from build123d import *

# Parameters (mm, degrees)
PAD005_DEPTH                  = 17
PAD006_DEPTH                  = 4.5
SKETCH015_R                   = 2.75
POCKET005_DEPTH               = 93.84909
SKETCH016_R                   = 5
POCKET006_DEPTH               = 16.5
PAD005_MIRRORED002_2_DEPTH    = 17
PAD006_MIRRORED002_2_DEPTH    = 4.5
SKETCH015_MIRRORED002_2_R     = 2.75
POCKET005_MIRRORED002_2_DEPTH = 93.84909
SKETCH016_MIRRORED002_2_R     = 5
POCKET006_MIRRORED002_2_DEPTH = 16.5
SKETCH023_W                   = 1
SKETCH023_H                   = 10
POCKET011_DEPTH               = 0.2


with BuildPart() as part:
    # Sketch013 → Pad005 (new body)
    with BuildSketch(Plane.YZ):
        with BuildLine():
            ThreePointArc((0, -13.5), (4.330629, -12.786542), (8.203522, -10.721578))
            ThreePointArc((10.083563, -12.5), (9.900722, -10.810344), (8.203522, -10.721578))
            Line((6, -18.5), (10.083563, -12.5))
            Line((0, -18.5), (6, -18.5))
            Line((0, -13.5), (0, -18.5))
        make_face()
    pad005 = extrude(amount=PAD005_DEPTH)

    # Sketch014 → Pad006 (join)
    with BuildSketch(Plane.YZ.offset(17)):
        with BuildLine():
            ThreePointArc((0, -10.15), (8.790158, -5.075), (8.790158, 5.075))
            ThreePointArc((12.773875, 11.975), (8.790158, 9.675), (8.790158, 5.075))
            ThreePointArc((12.773875, 9.125), (14.198875, 10.55), (12.773875, 11.975))
            ThreePointArc((12.773875, 9.125), (11.25833, 8.25), (11.25833, 6.5))
            ThreePointArc((12.442941, -3.764734), (12.914285, 1.490384), (11.25833, 6.5))
            Line((12.442941, -3.764734), (9.8, -12.5))
            Line((9.8, -12.5), (0, -14.15))
            Line((0, -10.15), (0, -14.15))
        make_face()
    pad006 = extrude(amount=-PAD006_DEPTH)

    # Sketch015 → Pocket005 (cut, through all)
    with BuildSketch(Plane.XY):
        Circle(SKETCH015_R)
    pocket005 = extrude(amount=-POCKET005_DEPTH, mode=Mode.SUBTRACT)

    # Sketch016 → Pocket006 (cut)
    with BuildSketch(Plane.XY):
        Circle(SKETCH016_R)
    pocket006 = extrude(amount=-POCKET006_DEPTH, mode=Mode.SUBTRACT)

    # Sketch013 Mirrored002 2 → Pad005 Mirrored002 2 (add)
    with BuildSketch(Plane(origin=(0, 0, 0), x_dir=(0, -1, 0), z_dir=(-1, 0, 0))):
        with BuildLine():
            ThreePointArc((0, -13.5), (4.330629, -12.786542), (8.203522, -10.721578))
            ThreePointArc((10.083563, -12.5), (9.900722, -10.810344), (8.203522, -10.721578))
            Line((6, -18.5), (10.083563, -12.5))
            Line((0, -18.5), (6, -18.5))
            Line((0, -13.5), (0, -18.5))
        make_face()
    pad005_mirrored002_2 = extrude(amount=-PAD005_MIRRORED002_2_DEPTH)

    # Sketch014 Mirrored002 2 → Pad006 Mirrored002 2 (add)
    with BuildSketch(Plane(origin=(17, 0, 0), x_dir=(0, -1, 0), z_dir=(-1, 0, 0))):
        with BuildLine():
            ThreePointArc((0, -10.15), (8.790158, -5.075), (8.790158, 5.075))
            ThreePointArc((12.773875, 11.975), (8.790158, 9.675), (8.790158, 5.075))
            ThreePointArc((12.773875, 9.125), (14.198875, 10.55), (12.773875, 11.975))
            ThreePointArc((12.773875, 9.125), (11.25833, 8.25), (11.25833, 6.5))
            ThreePointArc((12.442941, -3.764734), (12.914285, 1.490384), (11.25833, 6.5))
            Line((12.442941, -3.764734), (9.8, -12.5))
            Line((9.8, -12.5), (0, -14.15))
            Line((0, -10.15), (0, -14.15))
        make_face()
    pad006_mirrored002_2 = extrude(amount=PAD006_MIRRORED002_2_DEPTH)

    # Sketch015 Mirrored002 2 → Pocket005 Mirrored002 2 (cut, through all)
    with BuildSketch(Plane(origin=(0, 0, 0), x_dir=(1, 0, 0), z_dir=(0, 0, -1))):
        Circle(SKETCH015_MIRRORED002_2_R)
    pocket005_mirrored002_2 = extrude(amount=POCKET005_MIRRORED002_2_DEPTH, mode=Mode.SUBTRACT)

    # Sketch016 Mirrored002 2 → Pocket006 Mirrored002 2 (cut)
    with BuildSketch(Plane(origin=(0, 0, 0), x_dir=(1, 0, 0), z_dir=(0, 0, -1))):
        Circle(SKETCH016_MIRRORED002_2_R)
    pocket006_mirrored002_2 = extrude(amount=POCKET006_MIRRORED002_2_DEPTH, mode=Mode.SUBTRACT)

    # Mirrored003: Pad005, Pad006, Pocket005, Pocket006, Pad005 Mirrored002 2, Pad006 Mirrored002 2, Pocket005 Mirrored002 2, Pocket006 Mirrored002 2 across YZ
    add(pad005.mirror(Plane.YZ))
    add(pad006.mirror(Plane.YZ))
    add(pocket005.mirror(Plane.YZ), mode=Mode.SUBTRACT)
    add(pocket006.mirror(Plane.YZ), mode=Mode.SUBTRACT)
    add(pad005_mirrored002_2.mirror(Plane.YZ))
    add(pad006_mirrored002_2.mirror(Plane.YZ))
    add(pocket005_mirrored002_2.mirror(Plane.YZ), mode=Mode.SUBTRACT)
    add(pocket006_mirrored002_2.mirror(Plane.YZ), mode=Mode.SUBTRACT)

    # Sketch023 → Pocket011 (cut)
    with BuildSketch(Plane.YZ.offset(29)):
        with Locations((0, -15)):
            Rectangle(SKETCH023_W, SKETCH023_H)
    pocket011 = extrude(amount=-POCKET011_DEPTH, mode=Mode.SUBTRACT)

    # Mirrored006: Pocket011 across YZ
    add(pocket011.mirror(Plane.YZ), mode=Mode.SUBTRACT)


solid = part.part
Build history of the part. All positions in model axes, mm. A direction names the side the tool comes from. Coordinates: 2 decimals unless noted, no trailing zeros. Order: outer loops, then holes, each group sorted by start corner. A loop starts at its lowest first (then second) coordinate and runs counter-clockwise, first axis right, second up. Notation, with made-up numbers: (71.25, -17.5) - (106.25, -17.5) arc R20 ccw to (106.25, -7.5) - close; hole circle Ø7 at (69.25, 3.5). An arc over 180 degrees is marked (long way). Write each question's results on one line, items separated by ' | '. Start each with the question number.
Item 1: Tool access for faces 4 (the face through (0.24, -9.92, -10.83)), 5 (the face through (-2.685, 0.596, -17.486)), 6 (the face through (14.782, 8.824, 9.733)), 7 (the face through (-12.5, -6.4, -8.3)): list every direction of +Z, -Z, +X, -X, +Y, -Y with a clear straight run to the whole face (end or side of a thin tool).
Item 2: Band-saw the part on A-A on x = 11. Write the cut outline in (y, z).
Item 3: Band-saw the part on D-D on z = 4.5. Write the cut outline in (x, y), and give its area (3 significant figures).
Item 4: Wall check: probe 1 along X at (y, z) = (0, -13.75); probe 2 along X at (y, z) = (9, -8); probe 3 along Z at (x, y) = (8.5, 0.5). Give the ranges that are in metal, low to high. Write a range as [from, to].
Item 5: Band-saw the part on B-B on z = -6. Write the cut outline in (x, y).
Item 6: Band-saw the part on C-C on y = 7.5. Write the cut outline in (x, z).
Item 7: Mould opens along Z. For faces 1 (the face through (0.238, -8.013, -15.542)), 2 (the face through (12.5, -6.4, -8.3)), 3 (the face through (14.782, -12.923, 1.416)) say: released by +Z, released by -Z, zero draft, split by the parting line, or undercut.
Item 8: Flat gauge pins, fed straight in: pin 1 (6 mm diameter, centred on x = -13, z = -2.5, fed in from +Y); pin 2 (3 mm diameter, centred on x = -2, y = 0.5, fed in from +Z); pin 3 (5.5 mm diameter, centred on x = -3, y = -3, fed in from +Z). Where does each tip first touch, or does it go through?
Numbers:
1) face 4: none | face 5: +Z, -Z | face 6: +X, -X | face 7: +Z
2) outline: (-10.08, -12.5) - (-6, -18.5) - (6, -18.5) - (10.08, -12.5) arc R1.31 ccw to (8.2, -10.72) arc R13.5 cw to (-8.2, -10.72) arc R1.31 ccw to start
3) outline: (-17, -12.2) - (-12.5, -12.2) - (-12.5, -9.1) - (-17, -9.1) - close; (-17, 9.1) - (-12.5, 9.1) - (-12.5, 12.2) - (-17, 12.2) - close; (12.5, -12.2) - (17, -12.2) - (17, -9.1) - (12.5, -9.1) - close; (12.5, 9.1) - (17, 9.1) - (17, 12.2) - (12.5, 12.2) - close | area: 55.8 mm^2
4) probe 1: [-17, -5], [5, 17] | probe 2: [-17, -12.5], [12.5, 17] | probe 3: [-18.5, -13.49]
5) outline: (-17, -11.77) - (-12.5, -11.77) - (-12.5, -8.19) - (-17, -8.19) - close; (-17, 8.19) - (-12.5, 8.19) - (-12.5, 11.77) - (-17, 11.77) - close; (12.5, -11.77) - (17, -11.77) - (17, -8.19) - (12.5, -8.19) - close; (12.5, 8.19) - (17, 8.19) - (17, 11.77) - (12.5, 11.77) - close
6) outline: (-17, -16.3) - (17, -16.3) - (17, -6.84) - (12.5, -6.84) - (12.5, -11.22) - (-12.5, -11.22) - (-12.5, -6.84) - (-17, -6.84) - close
7) face 1: released by -Z | face 2: zero draft | face 3: undercut
8) pin 1: y = 13 | pin 2: z = -16.5 | pin 3: z = -12.21
